Check sheet for the drawn part. Datum: minimum x, y, z corner. Units: mm. A direction names the side the tool comes from. Give positions to 0.01 mm unless a question says otherwise; leave off trailing zeros. Write each loop counter-clockwise with the first axis right and the second up, starting at its lowest first coordinate (ties: lowest second). Pieces come first, ordered by that corner, then holes. Notation, with made-up numbers: (-8, 55) -> (47, 55) arc R37 cw to (47, 94) -> close; hole circle Ø1 at (-14.75, 22.25). An arc over 180 degrees is marked (long way). Use CSV: the item, a comma, the result in double quotes. Start each with the question number.
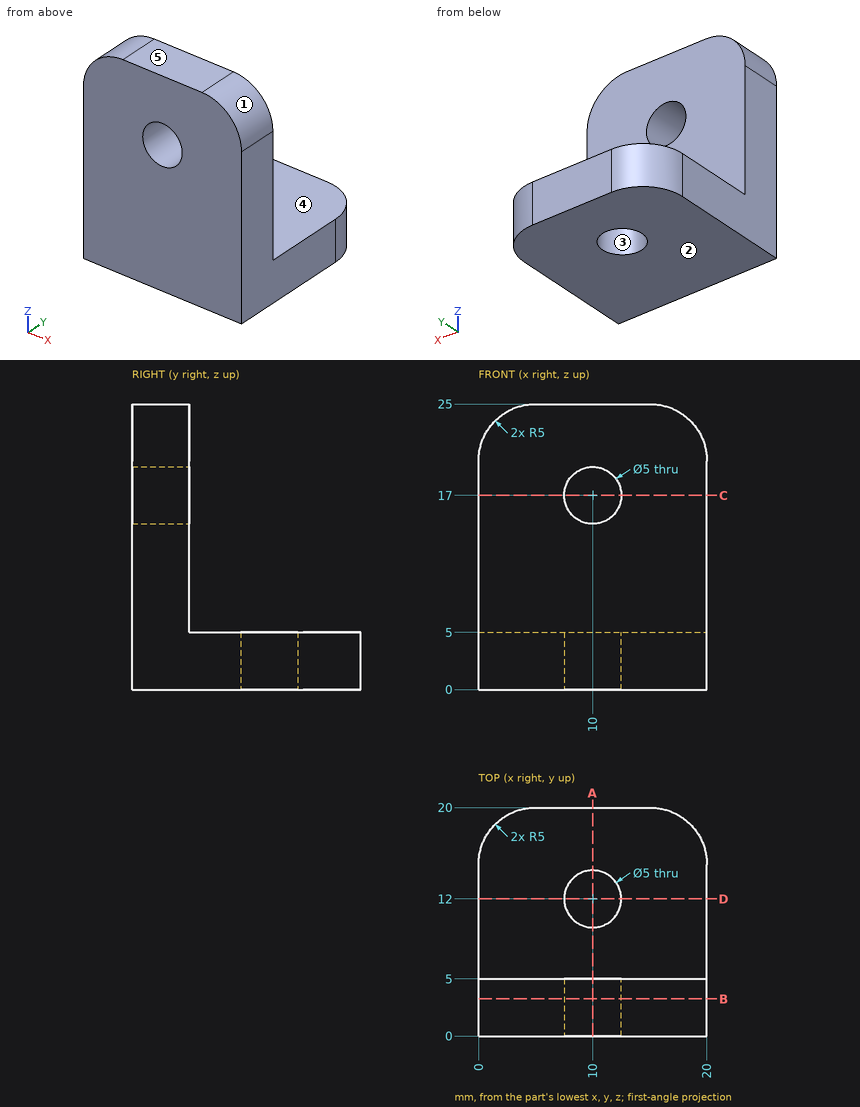
(1) Section check C-C on z = 17. Record the cut outline in (x, y), then the cut area to 3 significant figures.
(2) Go/stop test with flat-tipped pins: pin 1 (7.5 mm diameter, centred on x = 8, y = 11.5, fed in from +Z); pin 2 (4 mm diameter, centred on x = 17.5, y = 3, fed in from +Z); pin 3 (1.5 mm diameter, centred on x = 17, z = 16, fed in from +Y). Record where each tip stops, or that it passes through.
(3) Thickness scan on line 1 (Y direction, x = 10, z = 2); line 2 (Y direction, x = 18.5, z = 10.75); line 3 (Z direction, x = 10, y = 2.6). Record the ranges inside material, lowest first. Write a range as from..to.
(4) Section check A-A on x = 10. Record the cut outline in (y, z), then the cut area to 3 significant figures.
(5) Draft check along X on the marked faces 1, 2 and 3. Enter one of: released by +X, released by -X, zero draft, split by the parting line, or undercut.
(6) Set-up check for the marked faces 4 and 5: record each of +Z, -Z, +X, -X, +Y, -Y from which the full face is reachable in a straight line by a thin tool's end or side.
(7) Section check B-B on y = 3.25. Record the cut outline in (x, z), then the cut area to 3 significant figures.
Data:
1,outline,"(0, 0) -> (7.5, 0) -> (7.5, 5) -> (0, 5) -> close; (12.5, 0) -> (20, 0) -> (20, 5) -> (12.5, 5) -> close"
1,area,"75.0 mm2"
2,pin 1,"stops at z = 5"
2,pin 2,"stops at z = 24.97"
2,pin 3,"stops at y = 5"
3,line 1,"y = 0..9.5, 14.5..20"
3,line 2,"y = 0..5"
3,line 3,"z = 0..14.5, 19.5..25"
4,outline,"(0, 0) -> (9.5, 0) -> (9.5, 5) -> (5, 5) -> (5, 14.5) -> (0, 14.5) -> close; (0, 19.5) -> (5, 19.5) -> (5, 25) -> (0, 25) -> close; (14.5, 0) -> (20, 0) -> (20, 5) -> (14.5, 5) -> close"
4,area,"150 mm2"
5,face 1,"released by +X"
5,face 2,"zero draft"
5,face 3,"undercut"
6,face 4,"+Z, +X, -X, +Y"
6,face 5,"+Z, +X, -X, +Y, -Y"
7,outline,"(0, 0) -> (20, 0) -> (20, 20) arc R5 ccw to (15, 25) -> (5, 25) arc R5 ccw to (0, 20) -> close; hole circle Ø5 at (10, 17)"
7,area,"470 mm2"
